```python
from build123d import *

# Parameters (mm, degrees)
SALIENTE_EXTRUIR1_DEPTH = 6
REDONDEO1_R             = 5


with BuildPart() as part:
    # Croquis1 → Saliente-Extruir1 (new body)
    with BuildSketch(Plane.XY):
        with BuildLine():
            ThreePointArc((-5, 103.543560763), (0, 102.5), (5, 103.543560763))
            Line((5, 103.543560763), (5, 106.629665479))
            ThreePointArc((5, 106.629665479), (0, 105.25), (-5, 106.629665479))
            Line((-5, 106.629665479), (-5, 103.543560763))
        make_face()
        with BuildLine():
            Line((5, 106.629665479), (5, 103.543560763))
            ThreePointArc((5, 103.543560763), (10.458250332, 108.153468031), (12.5, 115))
            ThreePointArc((12.5, 115), (-6.846531969, 125.458250332), (-5, 103.543560763))
            Line((-5, 103.543560763), (-5, 106.629665479))
            ThreePointArc((-5, 106.629665479), (-4.812094139, 123.479755303), (9.75, 115))
            ThreePointArc((9.75, 115), (8.479755303, 110.187905861), (5, 106.629665479))
        make_face()
        with BuildLine():
            ThreePointArc((-5, 11.456439237), (0, 12.5), (5, 11.456439237))
            Line((5, 11.456439237), (5, 103.543560763))
            ThreePointArc((5, 103.543560763), (0, 102.5), (-5, 103.543560763))
            Line((-5, 103.543560763), (-5, 11.456439237))
        make_face()
        with BuildLine():
            ThreePointArc((-5, 8.370334521), (0, 9.75), (5, 8.370334521))
            Line((5, 8.370334521), (5, 11.456439237))
            ThreePointArc((5, 11.456439237), (0, 12.5), (-5, 11.456439237))
            Line((-5, 11.456439237), (-5, 8.370334521))
        make_face()
        with BuildLine():
            Line((5, 11.456439237), (5, 8.370334521))
            ThreePointArc((5, 8.370334521), (8.479755303, 4.812094139), (9.75, 0))
            ThreePointArc((9.75, 0), (-4.812094139, -8.479755303), (-5, 8.370334521))
            Line((-5, 8.370334521), (-5, 11.456439237))
            ThreePointArc((-5, 11.456439237), (-6.846531969, -10.458250332), (12.5, 0))
            ThreePointArc((12.5, 0), (10.458250332, 6.846531969), (5, 11.456439237))
        make_face()
    extrude(amount=SALIENTE_EXTRUIR1_DEPTH)

    # Redondeo1
    redondeo1_edges = [part.edges().sort_by_distance(p)[0] for p in [
        (-5, 11.456439237, 3),
        (-5, 103.543560763, 3),
        (5, 103.543560763, 3),
        (5, 11.456439237, 3),
    ]]
    fillet(redondeo1_edges, radius=REDONDEO1_R)


solid = part.part
```
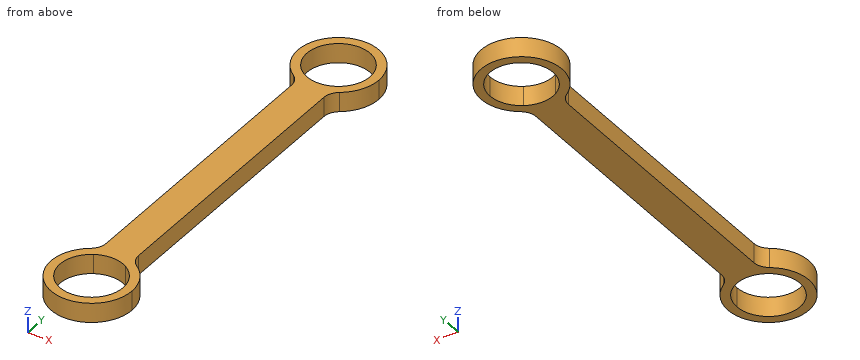
For this review, take the finished solid that the model builds, in its own axes (mm). Coordinates: 2 decimals unless noted, no trailing zeros. Order: outer loops, then holes, each group sorted by start corner. A loop starts at its lowest first (then second) coordinate and runs counter-clockwise, first axis right, second up. Notation, with made-up numbers: (87, -33) - (123, -33) arc R30 ccw to (123, -1) - close; hole circle Ø1 at (-8.75, 11). An arc over 180 degrees is marked (long way). Answer as a JSON object with one key per item and string values. Group by question number.
1. We need section D-D on y = 49.5. State the section outline as (x, z) points.
2. We need section B-B on x = 0. State the section outline as (y, z) points.
3. We need section C-C on y = 112. State the section outline as (x, z) points.
4. For probe 1 along Y at (x, z) = (0, 3.8); probe 2 along X at (y, z) = (115, 1.85); probe 3 along Y at (x, z) = (3.75, 4.75), list the stretches that pass through material, from the lowest coordinate up.
5. We need section A-A on z = 1.75. State the section outline as (x, y) points, then the cut area to 3 significant figures.
6. Clearance check with flat-ended pins moving along their axes: P1, Ø1, axis at x = 2.5, z = 5, coming from the -Y side; P2, Ø2, axis at x = -7, y = 47, coming from the -Z side; P3, Ø3, axis at y = 78, z = 2, coming from the -X side; P4, Ø3, axis at y = 66.5, z = 2.5, coming from the +X side. State where each tip first meets the part, or that it passes through.
Final values:
{
 "1": {"outline": "(-5, 0) - (5, 0) - (5, 6) - (-5, 6) - close"},
 "2": {"outline": "(-12.5, 0) - (-9.75, 0) - (-9.75, 6) - (-12.5, 6) - close; (9.75, 0) - (105.25, 0) - (105.25, 6) - (9.75, 6) - close; (124.75, 0) - (127.5, 0) - (127.5, 6) - (124.75, 6) - close"},
 "3": {"outline": "(-12.13, 0) - (-9.28, 0) - (-9.28, 6) - (-12.13, 6) - close; (9.28, 0) - (12.13, 0) - (12.13, 6) - (9.28, 6) - close"},
 "4": {"probe 1": "-12.5 to -9.75, 9.75 to 105.25, 124.75 to 127.5", "probe 2": "-12.5 to -9.75, 9.75 to 12.5", "probe 3": "-11.92 to -9, 9 to 106, 124 to 126.92"},
 "5": {"outline": "(-7.14, 10.26) arc R12.5 ccw (long way) to (7.14, 10.26) arc R5 cw to (5, 14.36) - (5, 100.64) arc R5 cw to (7.14, 104.74) arc R12.5 ccw (long way) to (-7.14, 104.74) arc R5 cw to (-5, 100.64) - (-5, 14.36) arc R5 cw to start; hole circle Ø19.5 at (0, 0); hole circle Ø19.5 at (0, 115)", "area": "1,300 mm²"},
 "6": {"P1": "y = -12.34", "P2": "through", "P3": "x = -5", "P4": "x = 5"}
}
